Input: part model. Units: mm. Frame: model coordinates. A direction names the side the tool comes from. Coordinates: 2 decimals unless noted, no trailing zeros. Write each loop counter-clockwise with the first axis right and the second up, starting at its lowest first coordinate (ties: lowest second). Pieces come first, ordered by that corner, then holes. Notation, with made-up numbers: (-37.5, -30.5) - (8.5, -30.5) arc R19 ccw to (8.5, 4.5) - close; hole circle Ø5 at (-11, -16.75). An arc over 180 degrees is marked (long way). Use CSV: the item, a comma, the result in double quotes.
Autodesk Inventor part; units mm, degrees
ref_plane "YZ Plane" through (0, 0, 0) normal (1, 0, 0) x (0, 1, 0)
ref_plane "XZ Plane" through (0, 0, 0) normal (0, 1, 0) x (-1, 0, 0)
ref_plane "XY Plane" through (0, 0, 0) normal (0, 0, 1) x (1, 0, 0)
sketch "Skizze1" plane through (0, 0, 0) normal (0, 1, 0) x (-1, 0, 0)
  line L0 (0, 0) -> (4, 0)
  line L1 (4, 0) -> (4, -10)
  line L2 (4, -10) -> (3, -10)
  line L3 (3, -10) -> (3, -19)
  line L4 (3, -19) -> (2.85, -19)
  line L5 (2.85, -19) -> (2.85, -19.8)
  line L6 (2.85, -19.8) -> (3, -19.8)
  line L7 (3, -19.8) -> (3, -22)
  line L8 (3, -22) -> (0, -22)
  line L9 (0, -22) -> (0, 0)
  point P0 (1.5, -22)
  dimension "d0" = 10
  dimension "d1" = 22
  dimension "d3" = 9
  dimension "d4" = 0.8
  dimension "d5" = 8
  dimension "d6" = 6
  dimension "d7" = 5.7
revolve "Umdrehung1" add sketch "Skizze1" angle 360 about axis through (0, 0, -22) along (0, 0, 1)
chamfer "Fasen1" distance 0.5 angle 45 1 edges at (3, 0, -22)
properties part number "Achse.planetenrad"
(1) Ray query, probe 1 along Z at (x, y) = (-0.5, 3); probe 2 along Z at (x, y) = (-2.5, -1.5); probe 3 along X at (y, z) = (2.25, -20). Return the intervals inside material, ascending. Write a range as from..to.
Check values:
probe 1,"-10..0"
probe 2,"-21.58..-19.8, -19..0"
probe 3,"-1.98..1.98"
(2) Cut plane A-A on x = 0. Return loops of the section in (y, z), and give its area (3 significant figures).
Check values:
outline,"(-4, -10) - (-3, -10) - (-3, -19) - (-2.85, -19) - (-2.85, -19.8) - (-3, -19.8) - (-3, -21.5) - (-2.5, -22) - (2.5, -22) - (3, -21.5) - (3, -19.8) - (2.85, -19.8) - (2.85, -19) - (3, -19) - (3, -10) - (4, -10) - (4, 0) - (-4, 0) - close"
area,"152 mm^2"
(3) Pin query (flat end, axial travel): pin 1 Ø3 at (x, z) = (2, -10) entering from -Y; pin 2 Ø4 at (x, z) = (1.5, -18.5) entering from +Y; pin 3 Ø4 at (y, z) = (-3, -7) entering from +X. Return the tip coordinate at first contact, or that it passes through.
Check values:
pin 1,"y = -3.97"
pin 2,"y = 3"
pin 3,"x = 3.87"
(4) Reachability of faces 5 (the cylindrical face through (0.867, -3.905, -5.07)), 6 (the flat face through (-1, -3, -10)) from +Z, -Z, +X, -X, +Y, -Y: full face, straight path, thin tool, end or side. Return the list, or none.
Check values:
face 5,"+Z, -Z"
face 6,"-Z"
(5) Cut plane C-C on z = -11.25. Return loops of the section in (x, y), and give its area (3 significant figures).
Check values:
outline,"circle Ø6 at (0, 0)"
area,"28.3 mm^2"
(6) Draft query along Z for faces 1 (the flat face through (0, 0, 0)), 2 (the cylindrical face through (2.262, -1.734, -19.406)), 3 (the flat face through (0, 0, -22)), 4 (the cylindrical face through (3, 0, -15)). Return one class per face: pulls with the +Z half, pulls with the -Z half, needs draft (parallel to the pull), parting line crosses it, or undercut.
Check values:
face 1,"pulls with the +Z half"
face 2,"undercut"
face 3,"pulls with the -Z half"
face 4,"needs draft"
(7) Cut plane D-D on x = 3.25. Return loops of the section in (y, z), and give its area (3 significant figures).
Check values:
outline,"(-2.33, -10) - (2.33, -10) - (2.33, 0) - (-2.33, 0) - close"
area,"46.6 mm^2"
